For this review, use the dimensioned drawing (mm, ordinates from the lowest corner) and the shaded views. A direction names the side the tool comes from. Round coordinates to 2 decimals unless told otherwise and drop trailing zeros. Write each loop counter-clockwise with the first axis right and the second up, starting at its lowest first coordinate (ties: lowest second). Pieces come first, ordered by that corner, then holes. Notation, with made-up numbers: M 53,-35 L 58,-35 A11 cw 58,-29 Z; hole C 73.25,42.25 d7. An arc over 180 degrees is marked long. One line per question, with ' | ' between items. Start each with the question number.
Item 1: Add section A-A, the plane y = 6. State the section outline as (x, z) points.
Item 2: Add section D-D, the plane y = 4.5. State the section outline as (x, z) points, and give its area (3 significant figures).
Item 3: Add section B-B, the plane x = 5.25. State the section outline as (y, z) points.
Item 4: For L1, parallel to Z at x = 7, y = 6.5; L2, parallel to X at y = 4.5, z = 9.25; L3, parallel to Z at x = 4.75, y = 1.5, list the stretches that pass through material, from the lowest coordinate up.
Item 5: Machinability: for the marked faces 1, 2, 3, 4 and 5, which of the approach directions +Z, -Z, +X, -X, +Y, -Y give a long, thin tool a straight path to every point of the face, cutting with its end or side? Answer none if there is none.
Item 6: Insertion check: pin 1 Ø3.5 at (x, y) = (4.5, 2) entering from +Z; pin 2 Ø2 at (x, z) = (4, 13) entering from -Y; pin 3 Ø2 at (y, z) = (2, 9) entering from +X; pin 4 Ø1.8 at (x, y) = (1.5, 4.5) entering from +Z. Each pin has a flat end and moves straight along its axis. Give the tip position at first contact, or say it passes through.
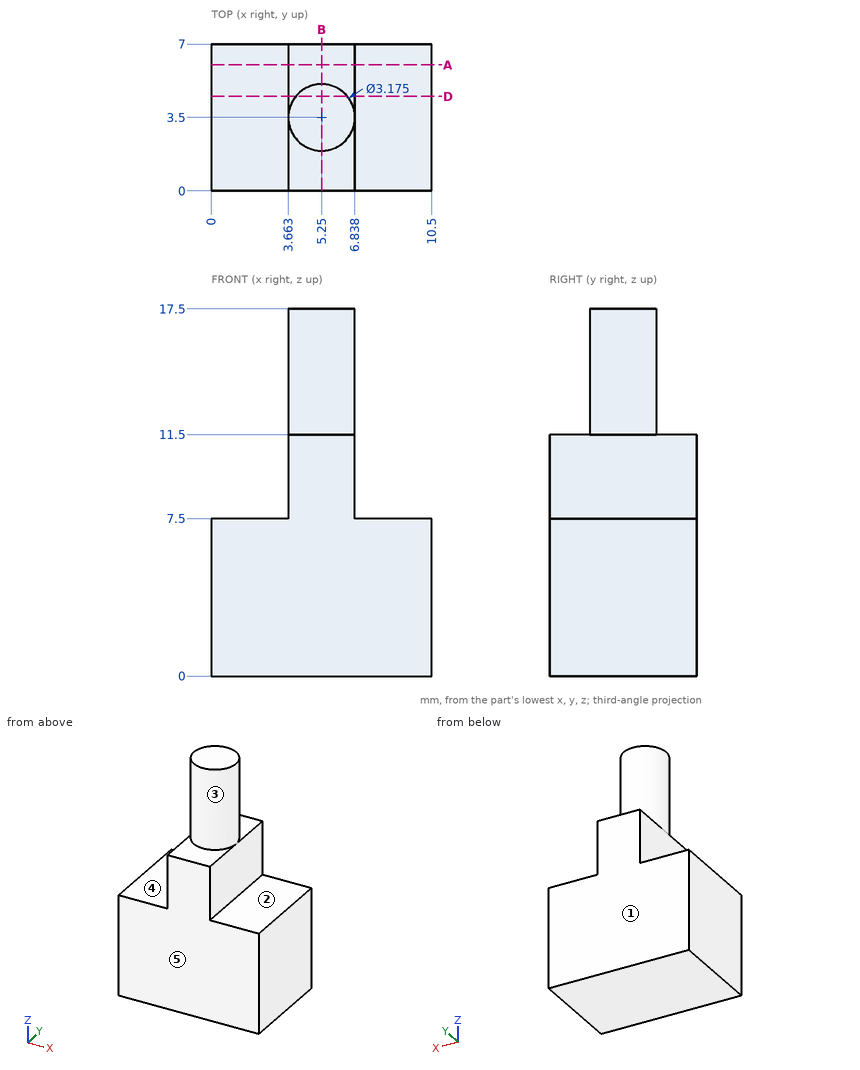
Computed values:
1) outline: M 0,0 L 10.5,0 L 10.5,7.5 L 6.84,7.5 L 6.84,11.5 L 3.66,11.5 L 3.66,7.5 L 0,7.5 Z
2) outline: M 0,0 L 10.5,0 L 10.5,7.5 L 6.84,7.5 L 6.84,11.5 L 6.48,11.5 L 6.48,17.5 L 4.02,17.5 L 4.02,11.5 L 3.66,11.5 L 3.66,7.5 L 0,7.5 Z | area: 106 mm^2
3) outline: M 0,0 L 7,0 L 7,11.5 L 5.09,11.5 L 5.09,17.5 L 1.91,17.5 L 1.91,11.5 L 0,11.5 Z
4) L1: z = 0 to 7.5 | L2: x = 3.66 to 6.84 | L3: z = 0 to 11.5
5) face 1: +Z, -Z, +X, -X, +Y | face 2: +Z, +X, +Y, -Y | face 3: +Z | face 4: +Z, -X, +Y, -Y | face 5: +Z, -Z, +X, -X, -Y
6) pin 1: stops at z = 17.5 | pin 2: stops at y = 1.93 | pin 3: stops at x = 6.84 | pin 4: stops at z = 7.5
